The drawing under review shows one solid part. Ordinate dimensions are in mm from its lowest x, y, z. A direction names the side the tool comes from. Round coordinates to 2 decimals unless told otherwise and drop trailing zeros. Order: outer loops, then holes, each group sorted by start corner. A loop starts at its lowest first (then second) coordinate and runs counter-clockwise, first axis right, second up. Notation, with made-up numbers: M 64,-14 L 119,-14 A14 cw 119,9 Z; hole C 6,-25.75 d2. An arc over 180 degrees is marked long. Answer as a JSON object with one key per item and string values. Group by question number.
1. To check wall thickness, follow probe 1 along Z at (x, y) = (24.5, 21); probe 2 along X at (y, z) = (24.5, 5). State the ranges of each line that lie inside material, in increasing order. Write a range as [from, to].
2. Add section A-A on y = 44.5. State the section outline as (x, z) points.
3. Add section B-B on x = 16.5. State the section outline as (y, z) points.
4. Machinability: for the marked faces 4 and 5, which of the approach directions +Z, -Z, +X, -X, +Y, -Y give a long, thin tool a straight path to every point of the face, cutting with its end or side? Answer none if there is none.
5. Clearance check with flat-ended pins moving along their axes: P1, Ø4, axis at x = 18.5, z = 26, coming from the -Y side; P2, Ø16.5, axis at x = 24.5, y = 38, coming from the -Z side; P3, Ø14, axis at x = 8, y = 33.5, coming from the -Z side. State where each tip first meets the part, or that it passes through.
6. Mouldability with a two-part tool opening along X and no side actions: class the marked faces 1, 2 and 3 as released by +X, released by -X, zero draft, split by the parting line, or undercut.
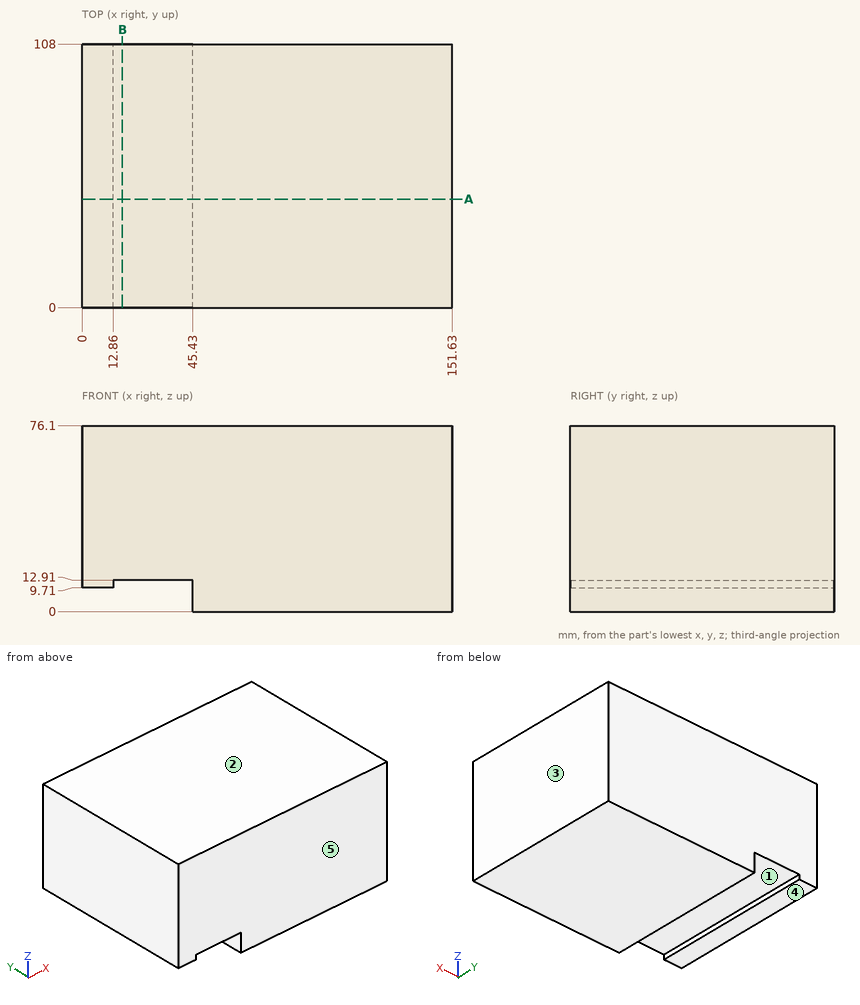
Recorded:
{
 "1": {"probe 1": "z = [12.91, 76.1]", "probe 2": "x = [45.43, 151.63]"},
 "2": {"outline": "M 0,9.71 L 12.86,9.71 L 12.86,12.91 L 45.43,12.91 L 45.43,0 L 151.63,0 L 151.63,76.1 L 0,76.1 Z"},
 "3": {"outline": "M 0,12.91 L 108,12.91 L 108,76.1 L 0,76.1 Z"},
 "4": {"face 4": "-Z, -X, +Y, -Y", "face 5": "+Z, -Z, +X, -X, -Y"},
 "5": {"P1": "stops at y = 0", "P2": "stops at z = 12.91", "P3": "stops at z = 9.71"},
 "6": {"face 1": "undercut", "face 2": "zero draft", "face 3": "released by +X"}
}
